Model file for the job. Use its own axes, mm. A direction names the side the tool comes from. Give positions to 0.01 mm unless a question says otherwise; leave off trailing zeros. Write each loop counter-clockwise with the first axis right and the second up, starting at its lowest first coordinate (ties: lowest second). Pieces come first, ordered by that corner, then holes. Notation, with made-up numbers: (13, -6) - (42, -6) arc R30 ccw to (42, 21) - close; hole circle Ø2 at (86.5, 11). An arc over 180 degrees is marked (long way). Use a Markdown table: item, result. Add a question column.
```python
from build123d import *

# Parameters (mm, degrees)
SKETCH1_W            = 115
SKETCH1_H            = 100
BOSS_EXTRUDE1_DEPTH  = 40
SKETCH8_R            = 7
SKETCH8_R_2          = 6
BOSS_EXTRUDE4_DEPTH  = 20
SKETCH9_W            = 200
SKETCH9_H            = 100
BOSS_EXTRUDE5_DEPTH  = 16.6
SKETCH10_R           = 9
SKETCH10_R_2         = 10
BOSS_EXTRUDE7_DEPTH  = 20
SKETCH17_W           = 15
SKETCH17_H           = 100
BOSS_EXTRUDE15_DEPTH = 20
SKETCH15_R           = 14.5
CUT_EXTRUDE2_DEPTH   = 10
SKETCH21_R           = 2
SKETCH21_R_2         = 6.075
CUT_EXTRUDE3_DEPTH   = 20
SKETCH28_W           = 100
SKETCH28_H           = 100
BOSS_EXTRUDE16_DEPTH = 20
SKETCH19_R           = 2
CUT_EXTRUDE4_DEPTH   = 40
SKETCH11_W           = 76.96
SKETCH11_H           = 72.932737716
SKETCH11_W_2         = 70.68
SKETCH11_H_2         = 66.981365666
SKETCH11_W_3         = 62.68
SKETCH11_H_3         = 59.4
BOSS_EXTRUDE17_DEPTH = 15
SKETCH35_W           = 15
SKETCH35_H           = 3
SKETCH35_W_2         = 3
SKETCH35_H_2         = 15
CUT_EXTRUDE14_DEPTH  = 3
SKETCH36_W           = 10
SKETCH36_H           = 48
CUT_EXTRUDE15_DEPTH  = 32
CUT_EXTRUDE16_DEPTH  = 3
FILLET1_R            = 3
SKETCH42_W           = 35
SKETCH42_H           = 66
CUT_EXTRUDE20_DEPTH  = 9
SKETCH43_R           = 2
CUT_EXTRUDE21_DEPTH  = 9
SKETCH45_W           = 10
SKETCH45_H           = 48
CUT_EXTRUDE22_DEPTH  = 32
CUT_EXTRUDE23_DEPTH  = 3
FILLET2_R            = 3
SKETCH47_W           = 35
SKETCH47_H           = 66
CUT_EXTRUDE24_DEPTH  = 9
SKETCH48_R           = 2
CUT_EXTRUDE25_DEPTH  = 9


with BuildPart() as part:
    # Sketch1 → Boss-Extrude1 (new body)
    with BuildSketch(Plane(origin=(0, 0, 0), x_dir=(1, 0, 0), z_dir=(0, 1, 0))):
        Rectangle(SKETCH1_W, SKETCH1_H)
    extrude(amount=BOSS_EXTRUDE1_DEPTH)

    # Sketch8 → Boss-Extrude4 (add)
    with BuildSketch(Plane.XZ):
        with Locations(Location((0, 0, 0), (0, 0, 90))):
            Circle(SKETCH8_R)
        with Locations(Location((42.407889557, -36.876425702, 0), (0, 0, 90))):
            Circle(SKETCH8_R_2)
        with Locations(Location((42.407889557, 36.876425702, 0), (0, 0, 90))):
            Circle(SKETCH8_R_2)
    extrude(amount=BOSS_EXTRUDE4_DEPTH)

    # Sketch9 → Boss-Extrude5 (add)
    with BuildSketch(Plane.XZ.offset(20)):
        with Locations((-42.5, 0)):
            Rectangle(SKETCH9_W, SKETCH9_H)
    extrude(amount=BOSS_EXTRUDE5_DEPTH)

    # Sketch10 → Boss-Extrude7 (add)
    with BuildSketch(Plane.XZ.offset(36.6)):
        with Locations(Location((37.5, -25, 0), (0, 0, 270))):
            Circle(SKETCH10_R)
        with Locations(Location((-122.5, -25, 0), (0, 0, 90))):
            Circle(SKETCH10_R)
        with Locations(Location((-122.5, 25, 0), (0, 0, 270))):
            Circle(SKETCH10_R)
        with Locations(Location((37.5, 25, 0), (0, 0, 90))):
            Circle(SKETCH10_R)
        with Locations(Location((-42.5, 0, 0), (0, 0, 270))):
            Circle(SKETCH10_R_2)
    extrude(amount=BOSS_EXTRUDE7_DEPTH)

    # Sketch17 → Boss-Extrude15 (add)
    with BuildSketch(Plane.XZ):
        with Locations((-50, 0)):
            Rectangle(SKETCH17_W, SKETCH17_H)
    extrude(amount=BOSS_EXTRUDE15_DEPTH)

    # Sketch15 → Cut-Extrude2 (cut)
    with BuildSketch(Plane(origin=(0, -20, 0), x_dir=(1, 0, 0), z_dir=(0, 1, 0))):
        with Locations(Location((-79, 0, 0), (0, 0, 270))):
            Circle(SKETCH15_R)
    extrude(amount=-CUT_EXTRUDE2_DEPTH, mode=Mode.SUBTRACT)

    # Sketch21 → Cut-Extrude3 (cut)
    with BuildSketch(Plane(origin=(0, -30, 0), x_dir=(1, 0, 0), z_dir=(0, 1, 0))):
        with Locations(Location((-90, 0, 0), (0, 0, 270))):
            Circle(SKETCH21_R)
        with Locations(Location((-68, 0, 0), (0, 0, 270))):
            Circle(SKETCH21_R)
        with Locations(Location((-79, 0, 0), (0, 0, 270))):
            Circle(SKETCH21_R_2)
    extrude(amount=-CUT_EXTRUDE3_DEPTH, mode=Mode.SUBTRACT)

    # Sketch28 → Boss-Extrude16 (add)
    with BuildSketch(Plane.XZ):
        with Locations((7.5, 0)):
            Rectangle(SKETCH28_W, SKETCH28_H)
    extrude(amount=BOSS_EXTRUDE16_DEPTH)

    # Sketch19 → Cut-Extrude4 (cut)
    with BuildSketch(Plane.ZY.offset(57.5)):
        with Locations((-27.33, -16)):
            Circle(SKETCH19_R)
        with Locations((-27.33, 10)):
            Circle(SKETCH19_R)
        with Locations(Location((27.33, -16, 0), (0, 0, 180))):
            Circle(SKETCH19_R)
        with Locations(Location((27.33, 10, 0), (0, 0, 180))):
            Circle(SKETCH19_R)
    extrude(amount=-CUT_EXTRUDE4_DEPTH, mode=Mode.SUBTRACT)

    # Sketch11 → Boss-Extrude17 (add)
    # profile 1 of 2: a face of its own
    with BuildSketch(Plane(origin=(0, 40, 0), x_dir=(1, 0, 0), z_dir=(0, 1, 0))):
        Rectangle(SKETCH11_W, SKETCH11_H)
        Rectangle(SKETCH11_W_2, SKETCH11_H_2, mode=Mode.SUBTRACT)
    # profile 2 of 2: a face of its own
    with BuildSketch(Plane(origin=(0, 40, 0), x_dir=(1, 0, 0), z_dir=(0, 1, 0))):
        Rectangle(SKETCH11_W_3, SKETCH11_H_3)
    extrude(amount=BOSS_EXTRUDE17_DEPTH)

    # Sketch35 → Cut-Extrude14 (cut)
    with BuildSketch(Plane(origin=(0, 40, 0), x_dir=(1, 0, 0), z_dir=(0, 1, 0))):
        with Locations((-15.2, -31.590682833)):
            Rectangle(SKETCH35_W, SKETCH35_H)
        with Locations((-15.2, 31.590682833)):
            Rectangle(SKETCH35_W, SKETCH35_H)
        with Locations((15.2, -31.590682833)):
            Rectangle(SKETCH35_W, SKETCH35_H)
        with Locations((15.2, 31.590682833)):
            Rectangle(SKETCH35_W, SKETCH35_H)
        with Locations((-33.34, 15)):
            Rectangle(SKETCH35_W_2, SKETCH35_H_2)
        with Locations((-33.34, -15)):
            Rectangle(SKETCH35_W_2, SKETCH35_H_2)
        with Locations((33.34, 15)):
            Rectangle(SKETCH35_W_2, SKETCH35_H_2)
        with Locations((33.34, -15)):
            Rectangle(SKETCH35_W_2, SKETCH35_H_2)
    extrude(amount=-CUT_EXTRUDE14_DEPTH, mode=Mode.SUBTRACT)

    # Sketch36 → Cut-Extrude15 (cut)
    with BuildSketch(Plane.XY.offset(50)):
        with Locations((-34.5, 1.107079448)):
            Rectangle(SKETCH36_W, SKETCH36_H)
    extrude(amount=-CUT_EXTRUDE15_DEPTH, mode=Mode.SUBTRACT)

    # Sketch37 → Cut-Extrude16 (cut)
    with BuildSketch(Plane(origin=(-39.5, 0, 0), x_dir=(0, 0, -1), z_dir=(1, 0, 0))):
        Polygon((-29.206388375, 13.25), (-31.08277675, 10), (-29.206388375, 6.75), (-25.453611625, 6.75), (-23.57722325, 10), (-25.453611625, 13.25), align=None)
        Polygon((-29.206388375, -12.75), (-31.08277675, -16), (-29.206388375, -19.25), (-25.453611625, -19.25), (-23.57722325, -16), (-25.453611625, -12.75), align=None)
    extrude(amount=-CUT_EXTRUDE16_DEPTH, mode=Mode.SUBTRACT)

    # Fillet1
    fillet1_edges = [part.edges().sort_by_distance(p)[0] for p in [
        (-39.5, 1.107079448, 18),
        (-39.5, -22.892920552, 34),
        (-29.5, 1.107079448, 18),
        (-29.5, 25.107079448, 34),
        (-34.5, 25.107079448, 18),
        (-39.5, 25.107079448, 34),
        (-29.5, -22.892920552, 34),
    ]]
    fillet(fillet1_edges, radius=FILLET1_R)

    # Sketch42 → Cut-Extrude20 (cut)
    with BuildSketch(Plane.XY.offset(50)):
        with Locations((-34.5, 1.107079448)):
            Rectangle(SKETCH42_W, SKETCH42_H)
    extrude(amount=-CUT_EXTRUDE20_DEPTH, mode=Mode.SUBTRACT)

    # Sketch43 → Cut-Extrude21 (cut)
    with BuildSketch(Plane.XY.offset(41)):
        with Locations((-34.5, 28.107079448)):
            Circle(SKETCH43_R)
        with Locations((-24, 1.107079448)):
            Circle(SKETCH43_R)
        with Locations(Location((-34.5, -25.892920552, 0), (0, 0, 180))):
            Circle(SKETCH43_R)
        with Locations(Location((-45, 1.107079448, 0), (0, 0, 180))):
            Circle(SKETCH43_R)
    extrude(amount=-CUT_EXTRUDE21_DEPTH, mode=Mode.SUBTRACT)

    # Sketch45 → Cut-Extrude22 (cut)
    with BuildSketch(Plane(origin=(0, 0, -50), x_dir=(-1, 0, 0), z_dir=(0, 0, -1))):
        with Locations((34.5, 1.11)):
            Rectangle(SKETCH45_W, SKETCH45_H)
    extrude(amount=-CUT_EXTRUDE22_DEPTH, mode=Mode.SUBTRACT)

    # Sketch46 → Cut-Extrude23 (cut)
    with BuildSketch(Plane(origin=(-39.5, 0, 0), x_dir=(0, 0, -1), z_dir=(1, 0, 0))):
        Polygon((29.206388375, 13.25), (25.453611625, 13.25), (23.57722325, 10), (25.453611625, 6.75), (29.206388375, 6.75), (31.08277675, 10), align=None)
        Polygon((25.453611625, -12.75), (23.57722325, -16), (25.453611625, -19.25), (29.206388375, -19.25), (31.08277675, -16), (29.206388375, -12.75), align=None)
    extrude(amount=-CUT_EXTRUDE23_DEPTH, mode=Mode.SUBTRACT)

    # Fillet2
    fillet2_edges = [part.edges().sort_by_distance(p)[0] for p in [
        (-29.5, 1.11, -18),
        (-29.5, -22.89, -34),
        (-39.5, 1.11, -18),
        (-39.5, 25.11, -34),
        (-34.5, 25.11, -18),
        (-29.5, 25.11, -34),
        (-34.5, -22.89, -18),
        (-39.5, -22.89, -34),
    ]]
    fillet(fillet2_edges, radius=FILLET2_R)

    # Sketch47 → Cut-Extrude24 (cut)
    with BuildSketch(Plane(origin=(0, 0, -50), x_dir=(-1, 0, 0), z_dir=(0, 0, -1))):
        with Locations((34.5, 1.11)):
            Rectangle(SKETCH47_W, SKETCH47_H)
    extrude(amount=-CUT_EXTRUDE24_DEPTH, mode=Mode.SUBTRACT)

    # Sketch48 → Cut-Extrude25 (cut)
    with BuildSketch(Plane(origin=(0, 0, -41), x_dir=(-1, 0, 0), z_dir=(0, 0, -1))):
        with Locations((34.5, 28.11)):
            Circle(SKETCH48_R)
        with Locations((45, 1.11)):
            Circle(SKETCH48_R)
        with Locations(Location((24, 1.11, 0), (0, 0, 180))):
            Circle(SKETCH48_R)
        with Locations(Location((34.5, -25.89, 0), (0, 0, 180))):
            Circle(SKETCH48_R)
    extrude(amount=-CUT_EXTRUDE25_DEPTH, mode=Mode.SUBTRACT)


solid = part.part
```
(1) Probe probe 1 along Y at (x, z) = (-51, -27.33); probe 2 along X at (y, z) = (-33, 0) (3 decimals); probe 3 along X at (y, z) = (48, 2). List the from-to ranges inside material, lowest first. Write a range as [from, to].
(2) Band-saw the part on D-D (x = -129.5). Write the cut outline in (y, z), then the cut area to 3 significant figures.
(3) Two-plate mould, pull along Y, no slides. Class faces 5 (the flat face through (0, 55, 0)), 6 (the cylindrical face through (-130.09, -46.46, -20.16)), 7 (the flat face through (-34, -31.89, -46)): +Y half, -Y half, draft (parallel to the pull), parting line (faces both ways), or undercut.
(4) Band-saw the part on C-C (x = -20). Give the number of separate pieces and of enclosed holes in the cut face, then the cut area to 3 significant figures.
(5) Flat gauge pins, fed straight in: pin 1 (0.9 mm diameter, centred on x = -41.5, z = -27.5, fed in from -Y); pin 2 (10 mm diameter, centred on y = 9, z = -33.5, fed in from -X); pin 3 (1.5 mm diameter, centred on x = -41.5, z = 28, fed in from +Y). Where does each tip first touch, or does it go through?
(6) Band-saw the part on B-B (x = 12). Write the cut outline in (y, z).
(7) Which spindle directions (+Z, -Z, +X, -X, +Y, -Y) get a long thin tool onto all of the face, cutting with end or side? Do faces 1 (the cylindrical face through (-50.105, -17.352, 28.804)), 2 (the flat face through (-34, 28, -32)), 3 (the cylindrical face through (29.91, -46.46, 29.84)), 4 (the flat face through (-45, 1, 32)). Say none if no direction does.
(8) Band-saw the part on A-A (x = -90). Write the cut outline in (y, z).
Model answer:
| question | item | result |
|---|---|---|
| 1 | probe 1 | y = [-36.6, -18], [-14, 8], [12, 40] |
| 1 | probe 2 | x = [-142.5, -92], [-88, -85.075], [-72.925, -70], [-66, 57.5] |
| 1 | probe 3 | x = [-38.48, -35.34], [-31.34, 31.34], [35.34, 38.48] |
| 2 | outline | (-56.6, -30.66) - (-36.6, -30.66) - (-36.6, -50) - (-20, -50) - (-20, 50) - (-36.6, 50) - (-36.6, 30.66) - (-56.6, 30.66) - (-56.6, 19.34) - (-36.6, 19.34) - (-36.6, -19.34) - (-56.6, -19.34) - close |
| 2 | area | 2,110 mm^2 |
| 3 | face 5 | +Y half |
| 3 | face 6 | draft |
| 3 | face 7 | undercut |
| 4 | separate pieces | 1 |
| 4 | enclosed holes | 4 |
| 4 | area | 7,380 mm^2 |
| 5 | pin 1 | stops at y = -36.6 |
| 5 | pin 2 | stops at x = -57.5 |
| 5 | pin 3 | stops at y = 40 |
| 6 | outline | (-36.6, -50) - (40, -50) - (40, -36.47) - (55, -36.47) - (55, -33.49) - (40, -33.49) - (40, -33.09) - (37, -33.09) - (37, -30.09) - (40, -30.09) - (40, -29.7) - (55, -29.7) - (55, 29.7) - (40, 29.7) - (40, 30.09) - (37, 30.09) - (37, 33.09) - (40, 33.09) - (40, 33.49) - (55, 33.49) - (55, 36.47) - (40, 36.47) - (40, 50) - (-36.6, 50) - close |
| 7 | face 1 | -X |
| 7 | face 2 | -Z |
| 7 | face 3 | -Y |
| 7 | face 4 | +Z |
| 8 | outline | (-36.6, -50) - (-20, -50) - (-20, -9.45) - (-30, -9.45) - (-30, -2) - (-36.6, -2) - close; (-36.6, 2) - (-30, 2) - (-30, 9.45) - (-20, 9.45) - (-20, 50) - (-36.6, 50) - close |
